Autodesk Inventor part; units mm, degrees
ref_plane "YZ Plane" through (0, 0, 0) normal (1, 0, 0) x (0, 1, 0)
ref_plane "XZ Plane" through (0, 0, 0) normal (0, 1, 0) x (-1, 0, 0)
ref_plane "XY Plane" through (0, 0, 0) normal (0, 0, 1) x (1, 0, 0)
sketch "Sketch1" plane through (0, 0, 0) normal (0, 1, 0) x (-1, 0, 0)
  line L0 (17.3205, -10) -> (21.6506, -12.5)
  line L1 (0, 0) -> (25, 0) construction
  line L2 (17.3205, 10) -> (21.6506, 12.5)
  line L3 (-17.3205, -10) -> (-21.6506, -12.5)
  line L4 (-17.3205, 10) -> (-21.6506, 12.5)
  arc A0 (17.3205, 10) -> (-17.3205, 10) centre (0, 0) ccw
  arc A1 (-17.3205, -10) -> (17.3205, -10) centre (0, 0) ccw
  arc A2 (21.6506, 12.5) -> (-21.6506, 12.5) centre (0, 0) ccw
  arc A3 (-21.6506, -12.5) -> (21.6506, -12.5) centre (0, 0) ccw
  circle A4 centre (0, 0) radius 25
  point P0 (0, -20)
  point P1 (0, -20)
  dimension "d13" = 50
  dimension "d4" = 30
  dimension "d10" = 0
  dimension "d11" = 20
sketch "Sketch2" plane through (0, 0, 0) normal (0, 1, 0) x (-1, 0, 0)
  circle A0 centre (0, 0) radius 32.5
  dimension "d14" = 65
extrude "Extrusion1" add sketch "Sketch2" along normal blind 6.5
sketch "Sketch11" plane through (0, 6.5, 0) normal (0, 1, 0) x (1, 0, 0)
  line L0 (25, 10) -> (20, 10)
  line L1 (20, 10) -> (20, -20)
  line L2 (20, -20) -> (25, -20)
  line L3 (25, -20) -> (25, 10)
  line L4 (25, -20) -> (-25, -20)
  line L5 (-25, -20) -> (-25, -17.0323)
  line L6 (-25, -17.0323) -> (25, -17.0323)
  line L7 (25, -17.0323) -> (25, -20)
  line L8 (-25, -20) -> (-20, -20)
  line L9 (-20, -20) -> (-20, 10)
  line L10 (-20, 10) -> (-25, 10)
  line L11 (-25, 10) -> (-25, -20)
  circle A0 centre (0, 0) radius 32.5
  line L12 (20, 10) -> (29, 10)
  line L13 (29, 10) -> (29, 3)
  line L14 (29, 3) -> (20, 3)
  line L15 (20, 3) -> (20, 10)
  line L16 (0, 45) -> (0, 40)
  line L17 (-25, 10) -> (-20, 10)
  line L18 (-20, 10) -> (-20, -20)
  line L19 (-25, -20) -> (-25, 10)
  line L20 (-20, 10) -> (-29, 10)
  line L21 (-29, 10) -> (-29, 3)
  line L22 (-29, 3) -> (-20, 3)
  line L23 (-20, 3) -> (-20, 10)
  point P0 (0, -20)
  point P1 (20, -17.0323)
  point P2 (-20, -17.0323)
  point P3 (-25, 3)
  point P4 (25, 3)
  dimension "d79" = 30
  dimension "d80" = 50
  dimension "d81" = 5
  dimension "d82" = 5
  dimension "d83" = 30
  dimension "d85" = 25
  dimension "d86" = 25
  dimension "d87" = 20
  dimension "d90" = 9
  dimension "d91" = 7
  dimension "d92" = 9
  dimension "d118" = 40
extrude "Extrusion9" add sketch "Sketch11" along normal blind 20 contours L3 L14 L1 L0 | L12 L13 L14 L3 | L3 L6 L1 L14 | L3 L2 L1 L6 | L1 L4 L9 L6 | L9 L4 L5 L6 | L6 L11 L22 L9 | L22 L11 L10 L9 | L22 L21 L20 L11
sketch "Sketch12" plane through (-20, 6.5, -10) normal (0, 0, -1) x (-1, 0, 0)
  circle A0 centre (4, 5) radius 1.5
  line L0 (-14, -36) -> (-14, -31)
  line L1 (-14, -31) -> (-21, -31)
  circle A1 centre (4, 15) radius 1.5
  circle A2 centre (-44, 5) radius 1.5
  circle A3 centre (-44, 15) radius 1.5
  line L2 (9, 0) -> (9, 20)
  line L3 (12.5, 0) -> (-52.5, 0)
  point P0 (-20, -6.5)
  dimension "d93" = 3
  dimension "d96" = 10
  dimension "d99" = 48
  dimension "d102" = 5
  dimension "d103" = 5
extrude "Extrusion10" cut sketch "Sketch12" against normal blind 5.2
sketch "Sketch13" plane through (-25, 6.5, -3) normal (-1, 0, 0) x (0, 0, 1)
  line L0 (13, 1) -> (17, 1)
  line L1 (17, 1) -> (17, 51)
  line L2 (17, 51) -> (13, 51)
  line L3 (13, 51) -> (13, 1)
  line L4 (35.5, 0) -> (-29.5, 0)
  line L5 (23, 0) -> (23, 20)
  point P0 (3, -6.5)
  dimension "d108" = 50
  dimension "d109" = 1
  dimension "d110" = 6
  dimension "d111" = 4
extrude "Extrusion11" cut sketch "Sketch13" against normal blind 5.2
fillet "Fillet3" radius 2 9 edges at (-25, 16.5, 20) (25, 16.5, 20) (0, 6.5, 20) (25, 6.5, 8.5) (-25, 6.5, 8.5) (-29, 6.5, -6.5) (-27, 6.5, -3) (29, 6.5, -6.5) (27, 6.5, -3)
sketch "Sketch14" plane through (-23, 26.5, 20) normal (0, 0, 1) x (1, 0, 0)
  circle A0 centre (12.5, -10.5) radius 2.825
  line L0 (3, -20) -> (3, 0)
  line L1 (46, -18) -> (0, -18)
  point P0 (23, -26.5)
  dimension "d113" = 5.65
  dimension "d114" = 9.5
  dimension "d115" = 7.5
extrude "Extrusion12" cut sketch "Sketch14" against normal blind 10
sketch "Sketch15" plane through (0, 0, 0) normal (0, -1, 0) x (1, 0, 0)
  circle A0 centre (6.5, 0) radius 1.3
  circle A1 centre (14.6, 0) radius 1.3
  circle A2 centre (0, 6.5) radius 1.3
  circle A3 centre (0, 14.6) radius 1.3
  circle A4 centre (-6.5, 0) radius 1.3
  circle A5 centre (-14.6, 0) radius 1.3
  circle A6 centre (0, -6.5) radius 1.3
  circle A7 centre (0, -14.6) radius 1.3
  point P0 (0, 0)
  dimension "d119" = 2.6
  dimension "d120" = 2.6
  dimension "d121" = 6.5
  dimension "d122" = 8.1
  dimension "d125" = 360
extrude "Extrusion13" cut sketch "Sketch15" against normal blind 4
properties part number "rotacniZaklad"
Geometry: final body of the model. Coordinates: model frame, mm. A direction names the side the tool comes from. Give positions to 0.01 mm unless a question says otherwise; leave off trailing zeros. Order: outer loops, then holes, each group sorted by start corner. A loop starts at its lowest first (then second) coordinate and runs counter-clockwise, first axis right, second up. Notation, with made-up numbers: (24, 33.5) -> (46, 33.5) arc R30 ccw to (46, 62.5) -> close; hole circle Ø7 at (83, 5.5). An arc over 180 degrees is marked (long way). Write each question's results on one line, items separated by ' | '.
1) Cut plane B-B (y = 16). Output: boundary loops of the cut face in (x, z) (3 decimals).
Geometry says:
outline: (-29, -10) -> (-20, -10) -> (-20, 10) -> (-25, 10) -> (-25, -3) -> (-29, -3) -> close; (-25, 14) -> (-20, 14) -> (-20, 17.032) -> (-13.325, 17.032) -> (-13.325, 20) -> (-23, 20) arc R2 ccw to (-25, 18) -> close; (-7.675, 17.032) -> (20, 17.032) -> (20, -10) -> (29, -10) -> (29, -3) -> (25, -3) -> (25, 18) arc R2 ccw to (23, 20) -> (-7.675, 20) -> close
2) Draft query along Y for faces 5 (the face through (24.43, 17.37, 19.4)), 6 (the face through (15, 4, 0)), 7 (the face through (29.6, 7.07, -6.56)), 8 (the face through (-22.89, 22.51, -7.44)). Return one class per face: released by +Y, released by -Y, zero draft, split by the parting line, or undercut.
Geometry says:
face 5: zero draft | face 6: released by -Y | face 7: released by +Y | face 8: undercut
3) Line query: line 1 along Z through (x, y) = (0, 1.5); line 2 along X through (y, z) = (18.5, 6.5); line 3 along Z through (x, y) = (-27, 20.25). Output: solid intervals per line, ascending.
Geometry says:
line 1: z = -32.5 to -15.9, -13.3 to -7.8, -5.2 to 5.2, 7.8 to 13.3, 15.9 to 32.5 | line 2: x = -25 to -20, 20 to 25 | line 3: z = -10 to -3
4) Cut plane C-C (z = -6.5). Output: boundary loops of the cut face in (x, y).
Geometry says:
outline: (-31.84, 0) -> (-1.3, 0) -> (-1.3, 4) -> (1.3, 4) -> (1.3, 0) -> (31.84, 0) -> (31.84, 6.5) -> (31, 6.5) arc R2 cw to (29, 8.5) -> (29, 26.5) -> (20, 26.5) -> (20, 6.5) -> (-20, 6.5) -> (-20, 26.5) -> (-29, 26.5) -> (-29, 8.5) arc R2 cw to (-31, 6.5) -> (-31.84, 6.5) -> close; hole circle Ø3 at (-24, 11.5); hole circle Ø3 at (-24, 21.5); hole circle Ø3 at (24, 11.5); hole circle Ø3 at (24, 21.5)
5) First-contact query: pin 1 Ø2.5 at (x, z) = (-6.5, 0) entering from +Y; pin 2 Ø5 at (x, y) = (-24, 15) entering from -Z; pin 3 Ø0.8 at (x, z) = (-0.5, -7) entering from -Y. Flat tips, straight axial feed; report the tip coordinate or a pass-through.
Geometry says:
pin 1: stops at y = 6.5 | pin 2: stops at z = -10 | pin 3: stops at y = 4
6) Cut plane A-A (y = 21.5). Output: boundary loops of the cut face in (x, z), and give its area (3 significant figures).
Geometry says:
outline: (-29, -10) -> (-25.5, -10) -> (-25.5, -4.8) -> (-22.5, -4.8) -> (-22.5, -10) -> (-20, -10) -> (-20, 10) -> (-25, 10) -> (-25, -3) -> (-29, -3) -> close; (-25, 14) -> (-20, 14) -> (-20, 17.03) -> (20, 17.03) -> (20, -10) -> (22.5, -10) -> (22.5, -4.8) -> (25.5, -4.8) -> (25.5, -10) -> (29, -10) -> (29, -3) -> (25, -3) -> (25, 18) arc R2 ccw to (23, 20) -> (-23, 20) arc R2 ccw to (-25, 18) -> close | area: 422 mm²
7) Cut plane D-D (x = -17.5). Output: boundary loops of the cut face in (y, z), and give its area (3 significant figures).
Geometry says:
outline: (0, -27.39) -> (6.5, -27.39) -> (6.5, 17.03) -> (26.5, 17.03) -> (26.5, 20) -> (8.5, 20) arc R2 cw to (6.5, 22) -> (6.5, 27.39) -> (0, 27.39) -> close | area: 416 mm²
8) Set-up query: faces 1 (the face through (-20, 16, 4)), 2 (the face through (-0.17, 1.97, -13.31)), 3 (the face through (29, 17, -7)), 4 (the face through (-25.6, 7.07, 7.65)). Return all of +Z, -Z, +X, -X, +Y, -Y with unobstructed straight access to the full face (end or side cutting, diameter ignored); none if empty.
Geometry says:
face 1: -Z, +Y | face 2: -Y | face 3: +Z, -Z, +X, +Y | face 4: +Z, -X, +Y
